Input: part model. Units: mm. Frame: model coordinates. Round coordinates to 2 decimals unless told otherwise and drop trailing zeros. Loops run counter-clockwise (first coordinate to the right, second up) from the corner with the lowest first, then second, coordinate; pieces in that order, holes last. Notation, with made-up numbers: (61, 63.25) -> (97, 63.25) arc R18 cw to (97, 76.25) -> close; hole circle Ø2 at (66.5, 42). An arc over 180 degrees is marked (long way). Answer as a JSON object with one key per item and string values. Group by question number.
Item 1: Material intervals for line 1 (X direction, y = 23.5, z = 5.5); line 2 (X direction, y = -109, z = -2.5); line 3 (Y direction, x = 462, z = -1.5), sorted ascending. Write a range as [from, to].
Item 2: Pin query (flat end, axial travel): pin 1 (4 mm diameter, centred on y = 154.5, z = -8, fed in from +X); pin 2 (12 mm diameter, centred on x = 222.5, y = 310.5, fed in from +Z); pin 3 (4 mm diameter, centred on x = 466, z = 2.5, fed in from +Y); pin 4 (1 mm diameter, centred on x = 262.5, z = -2, fed in from -Y). Return the tip coordinate at first contact, or that it passes through.
Item 3: Section query A-A on z = 5. Return loops of the section in (x, y), and give its area (3 significant figures).
from build123d import *


with BuildPart() as f2:
    # F2: sweep along a path in F1
    with BuildLine(Plane.XY) as f2_path:
        CenterArc((431.5, 0), 412.5, 0, 360)
    # F0 (on Front) → F2 (sweep)
    with BuildSketch(Plane.XZ):
        with BuildLine():
            Line((0, 8), (0, 0))
            Line((0, 0), (38, 0))
            Line((38, 0), (42.4131194186, -10.4150611426))
            Line((42.4131194186, -10.4150611426), (42.8641578953, -10.4150611426))
            ThreePointArc((42.8641578953, -10.4150611426), (47.0327096225, -8.1760711929), (47.467923181, -3.4643317419))
            Line((47.467923181, -3.4643317419), (46, 0))
            Line((46, 0), (45.194304801, 1.9014588014))
            ThreePointArc((45.194304801, 1.9014588014), (41.5087943304, 6.3371034543), (35.9867742297, 8))
            Line((35.9867742297, 8), (0, 8))
        make_face()
    sweep(path=f2_path.line)


solid = f2.part
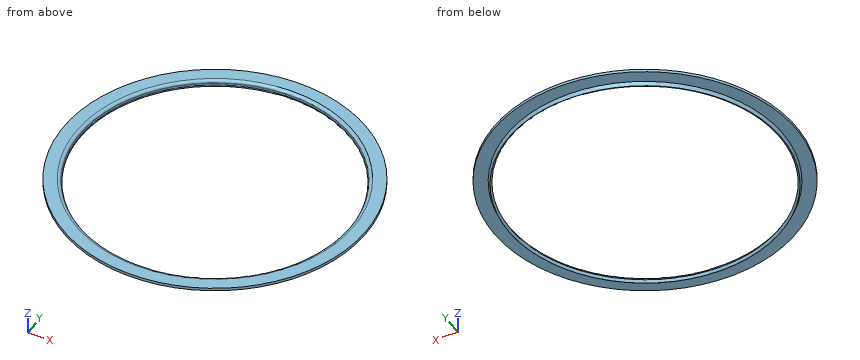
Solved:
{
 "1": {"line 1": "[0.64, 43.31], [819.69, 862.36]", "line 2": "[54.5, 62.84], [800.16, 808.5]", "line 3": "[-391.68, -383.65], [383.65, 391.68]"},
 "2": {"pin 1": "x = 790.97", "pin 2": "through", "pin 3": "y = 430.27", "pin 4": "y = -354.76"},
 "3": {"outline": "circle Ø863 at (431.5, 0); hole circle Ø776.74 at (431.5, 0)", "area": "111,000 mm²"}
}
